Work out the finished part from the listing and answer in its coordinate system (mm). Face numbers are marked on the shaded views. Coordinates: 2 decimals unless noted, no trailing zeros. Write each loop counter-clockwise with the first axis right and the second up, starting at its lowest first coordinate (ties: lowest second). Pieces come first, ordered by that corner, then holes. Notation, with made-up numbers: (-33, 74.5) - (-19, 74.5) arc R20 cw to (-19, 107.5) - close; hole circle Ø10 at (-15, -6.5). An arc over 180 degrees is marked (long way). Use a Markdown table: item, result. Add a question column.
(1) The part is cut by section D-D, the plane x = -61. Give the vertices of the cut face in (y, z), then the cut area to 3 significant figures.
(2) Given pin 1 Ø21.5 at (x, z) = (32.5, -14) entering from +Y; pin 2 Ø1.6 at (x, y) = (-78.95, 4) entering from +Z; pin 3 Ø1.5 at (x, y) = (33.5, -4) entering from +Z; pin 4 Ø4 at (x, y) = (31.5, 1.5) entering from -Z, each flat-ended and moving along its own axis, determine where each tip first touches the part or whether it passes through.
(3) For a pull along X with two mould halves and no side action, classify the marked faces 1, 2 and 3 as released by +X, released by -X, zero draft, split by the parting line, or undercut.
(4) The part is cut by section C-C, the plane y = -3.25. Give the vertices of the cut face in (x, z).
(5) Find the intervals of material crossed by line 1 (Z direction, x = -43.5, y = -3); line 2 (X direction, y = -2.75, z = 21); line 3 (X direction, y = -2, z = 18), in increasing order. Write a range as from..to.
(6) The part is cut by section B-B, the plane z = 29.5. Give the vertices of the cut face in (x, y).
(7) The part is cut by section A-A, the plane x = 44. Give the vertices of the cut face in (y, z), then the cut area to 3 significant figures.
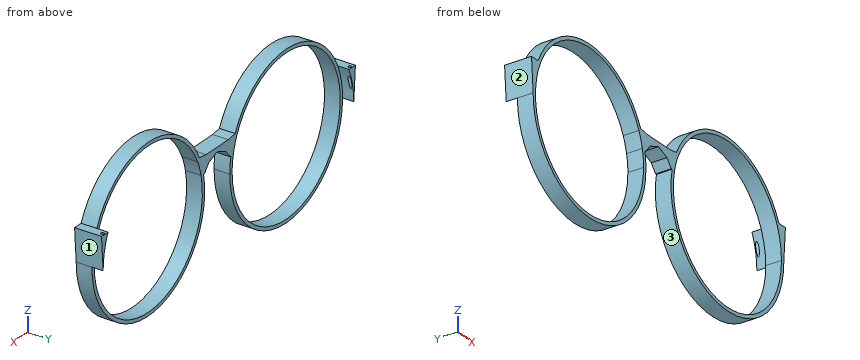
from build123d import *

# Parameters (mm, degrees)
F1_DEPTH = 7
F2_DEPTH = 5
F3_R     = 0.7
F4_DEPTH = 36.001


# Not quite as in the source:
# - a feature names something its author has since deleted; it is built from what else it names


with BuildPart() as f1:
    # F0 (on Front) → F1 (new body)
    with BuildSketch(Plane.XZ):
        with BuildLine():
            ThreePointArc((76.8747497611, 14.6714289741), (44.3508342177, 35.9982904504), (11.4174388077, 15.3093666149))
            Line((11.4174388077, 15.3093666149), (12.4627336019, 13.9875240173))
            ThreePointArc((12.4627336019, 13.9875240173), (51.1489268169, 33.7511902807), (78.5, 0))
            ThreePointArc((78.5, 0), (40.255323539, -34.2961717718), (10.312904452, 7.4451053411))
            Line((10.312904452, 7.4451053411), (8.7300367759, 7.2131611772))
            ThreePointArc((8.7300367759, 7.2131611772), (40.3749949013, -35.8170258122), (80, 0))
            ThreePointArc((80, 0), (79.2100198197, 7.5003002806), (76.8747497611, 14.6714289741))
        make_face()
        with BuildLine():
            ThreePointArc((-10.312904452, 7.4451053411), (-9.7038282282, 3.744676461), (-9.5, 0))
            ThreePointArc((-9.5, 0), (-77.7511902807, -7.1489268169), (-12.4627336019, 13.9875240173))
            Line((-12.4627336019, 13.9875240173), (-11.4174388077, 15.3093666149))
            ThreePointArc((-11.4174388077, 15.3093666149), (-44.3508342177, 35.9982904504), (-76.8747497611, 14.6714289741))
            ThreePointArc((-76.8747497611, 14.6714289741), (-79.2100198197, 7.5003002806), (-80, 0))
            ThreePointArc((-80, 0), (-44, -36), (-8, 0))
            ThreePointArc((-8, 0), (-8.1829741878, 3.6250050987), (-8.7300367759, 7.2131611772))
            Line((-8.7300367759, 7.2131611772), (-10.312904452, 7.4451053411))
        make_face()
        with BuildLine():
            ThreePointArc((-12.4627336019, 13.9875240173), (-11.2241680754, 10.7700901411), (-10.312904452, 7.4451053411))
            Line((-10.312904452, 7.4451053411), (-8.7300367759, 7.2131611772))
            ThreePointArc((-8.7300367759, 7.2131611772), (-9.8330802816, 11.3411461924), (-11.4174388077, 15.3093666149))
            Line((-11.4174388077, 15.3093666149), (-12.4627336019, 13.9875240173))
        make_face()
        with BuildLine():
            ThreePointArc((-11.4174388077, 15.3093666149), (-9.8330802816, 11.3411461924), (-8.7300367759, 7.2131611772))
            Line((-8.7300367759, 7.2131611772), (-8.1688707932, 7.1309311988))
            Line((-8.1688707932, 7.1309311988), (-5.43964638, 10.5822112661))
            Line((-5.43964638, 10.5822112661), (-7.0639303873, 14.6714289741))
            Line((-7.0639303873, 14.6714289741), (-11.4174388077, 15.3093666149))
        make_face()
        Polygon((0, 14.6714289741), (-7.0639303873, 14.6714289741), (-5.43964638, 10.5822112661), (0, 12.7429009753), (5.43964638, 10.5822112661), (7.0639303873, 14.6714289741), align=None)
        with BuildLine():
            Line((11.4174388077, 15.3093666149), (7.0639303873, 14.6714289741))
            Line((7.0639303873, 14.6714289741), (5.43964638, 10.5822112661))
            Line((5.43964638, 10.5822112661), (8.1688707932, 7.1309311988))
            Line((8.1688707932, 7.1309311988), (8.7300367759, 7.2131611772))
            ThreePointArc((8.7300367759, 7.2131611772), (9.8330802816, 11.3411461924), (11.4174388077, 15.3093666149))
        make_face()
        with BuildLine():
            Line((12.4627336019, 13.9875240173), (11.4174388077, 15.3093666149))
            ThreePointArc((11.4174388077, 15.3093666149), (9.8330802816, 11.3411461924), (8.7300367759, 7.2131611772))
            Line((8.7300367759, 7.2131611772), (10.312904452, 7.4451053411))
            ThreePointArc((10.312904452, 7.4451053411), (11.2241680754, 10.7700901411), (12.4627336019, 13.9875240173))
        make_face()
        with BuildLine():
            Line((81.0259262548, 14.6714289741), (76.8747497611, 14.6714289741))
            ThreePointArc((76.8747497611, 14.6714289741), (79.2100198197, 7.5003002806), (80, 0))
            Line((80, 0), (81.0259262548, 14.6714289741))
        make_face()
        with BuildLine():
            ThreePointArc((-80, 0), (-79.2100198197, 7.5003002806), (-76.8747497611, 14.6714289741))
            Line((-76.8747497611, 14.6714289741), (-81.0259262548, 14.6714289741))
            Line((-81.0259262548, 14.6714289741), (-80, 0))
        make_face()
    extrude(amount=F1_DEPTH)

    # F0 (on Front) → F2 (join)
    with BuildSketch(Plane.XZ):
        with BuildLine():
            ThreePointArc((-80, 0), (-79.2100198197, 7.5003002806), (-76.8747497611, 14.6714289741))
            Line((-76.8747497611, 14.6714289741), (-81.0259262548, 14.6714289741))
            Line((-81.0259262548, 14.6714289741), (-80, 0))
        make_face()
        with BuildLine():
            Line((81.0259262548, 14.6714289741), (76.8747497611, 14.6714289741))
            ThreePointArc((76.8747497611, 14.6714289741), (79.2100198197, 7.5003002806), (80, 0))
            Line((80, 0), (81.0259262548, 14.6714289741))
        make_face()
    extrude(amount=-F2_DEPTH)

    # F3 (on Top) → F4 (cut, through all)
    with BuildSketch(Plane.XY):
        with Locations((-78.950338008, 4)):
            Circle(F3_R)
        with Locations((78.950338008, 4)):
            Circle(F3_R)
    extrude(amount=F4_DEPTH, mode=Mode.SUBTRACT)


solid = f1.part
Model answer:
| question | item | result |
|---|---|---|
| 1 | outline | (-7, -31.73) - (0, -31.73) - (0, -30.02) - (-7, -30.02) - close; (-7, 30.02) - (0, 30.02) - (0, 31.73) - (-7, 31.73) - close |
| 1 | area | 24.0 mm^2 |
| 2 | pin 1 | through |
| 2 | pin 2 | z = 14.67 |
| 2 | pin 3 | z = 34.65 |
| 2 | pin 4 | z = -34.22 |
| 3 | face 1 | released by +X |
| 3 | face 2 | released by -X |
| 3 | face 3 | undercut |
| 4 | outline | (-81.03, 14.67) - (-80, 0) arc R36 ccw (long way) to (-8.73, 7.21) - (-8.17, 7.13) - (-5.44, 10.58) - (0, 12.74) - (5.44, 10.58) - (8.17, 7.13) - (8.73, 7.21) arc R36 ccw (long way) to (80, 0) - (81.03, 14.67) - (76.87, 14.67) arc R36 ccw to (11.42, 15.31) - (7.06, 14.67) - (-7.06, 14.67) - (-11.42, 15.31) arc R36 ccw to (-76.87, 14.67) - close; hole circle Ø69 at (-44, 0); hole circle Ø69 at (44, 0) |
| 5 | line 1 | -36..-34.5, 34.5..36 |
| 5 | line 2 | -73.24..-71.37, -16.63..-14.76, 14.76..16.63, 71.37..73.24 |
| 5 | line 3 | -75.18..-73.43, -14.57..-12.82, 12.82..14.57, 73.43..75.18 |
| 6 | outline | (-64.63, -7) - (-61.89, -7) - (-61.89, 0) - (-64.63, 0) - close; (-26.11, -7) - (-23.37, -7) - (-23.37, 0) - (-26.11, 0) - close; (23.37, -7) - (26.11, -7) - (26.11, 0) - (23.37, 0) - close; (61.89, -7) - (64.63, -7) - (64.63, 0) - (61.89, 0) - close |
| 7 | outline | (-7, -36) - (0, -36) - (0, -34.5) - (-7, -34.5) - close; (-7, 34.5) - (0, 34.5) - (0, 36) - (-7, 36) - close |
| 7 | area | 21.0 mm^2 |
